Autodesk Inventor part; units mm, degrees
ref_plane "YZ Plane" through (0, 0, 0) normal (1, 0, 0) x (0, 1, 0)
ref_plane "XZ Plane" through (0, 0, 0) normal (0, 1, 0) x (-1, 0, 0)
ref_plane "XY Plane" through (0, 0, 0) normal (0, 0, 1) x (1, 0, 0)
sketch "Sketch1" plane through (0, 0, 0) normal (0, 0, 1) x (1, 0, 0)
  line L0 (-30, 30) -> (30, 30)
  line L1 (30, 30) -> (30, -30)
  line L2 (30, -30) -> (-30, -30)
  line L3 (-30, -30) -> (-30, 30)
  point P0 (0, 0)
  dimension "d0" = 60
  dimension "d1" = 60
  dimension "d2" = 30
  dimension "d3" = 30
extrude "Extrusion1" add sketch "Sketch1" along normal blind 2.6568
fillet "Fillet1" radius 2 2 edges at (30, -30, 1.3284) (-30, -30, 1.3284)
sketch "Sketch3" plane through (0, 0, 2.6568) normal (0, 0, 1) x (1, 0, 0)
  line L0 (-28, -30) -> (28, -30)
  line L1 (30, -28) -> (30, 30)
  line L2 (-30, 30) -> (-30, -28)
  line L3 (-15, -15) -> (-15, -25) construction
  line L4 (-17.75, -15) -> (-17.75, -25)
  line L5 (-12.25, -25) -> (-12.25, -15)
  arc A0 (-12.25, -15) -> (-17.75, -15) centre (-15, -15) ccw
  arc A1 (-17.75, -25) -> (-12.25, -25) centre (-15, -25) ccw
  line L6 (15, -15) -> (15, -25) construction
  line L7 (12.25, -15) -> (12.25, -25)
  line L8 (17.75, -25) -> (17.75, -15)
  arc A2 (17.75, -15) -> (12.25, -15) centre (15, -15) ccw
  arc A3 (12.25, -25) -> (17.75, -25) centre (15, -25) ccw
  point P0 (0, 0)
  point P1 (-15, -20)
  point P2 (15, -20)
  dimension "d14" = 10
  dimension "d15" = 5.5
  dimension "d16" = 5
  dimension "d17" = 15
  dimension "d18" = 5.5
  dimension "d19" = 45
  dimension "d20" = 10
  dimension "d21" = 5
extrude "Extrusion3" cut sketch "Sketch3" against normal through all
sketch "Sketch4" plane through (0, 0, 2.6568) normal (0, 0, 1) x (1, 0, 0)
  line L0 (30, -28) -> (30, 30)
  circle A0 centre (0, 9.85) radius 11
  line L1 (-28, -30) -> (28, -30)
  point P0 (0, 0)
  dimension "d24" = 22
  dimension "d25" = 30
  dimension "d31" = 39.85
extrude "Extrusion4" cut sketch "Sketch4" against normal blind 7
sketch "Sketch6" plane through (0, 0, 2.6568) normal (0, 0, 1) x (1, 0, 0)
  circle A0 centre (-15.5, -5.65) radius 1.75
  circle A1 centre (0, 9.85) radius 11
  point P0 (0, 0)
  dimension "d32" = 3.5
  dimension "d44" = 15.5
  dimension "d45" = 15.5
extrude "Extrusion6" cut sketch "Sketch6" against normal through all contours A0
pattern_linear "Rectangular Pattern1" count 2 spacing 31 along (1, 0, 0) count 2 spacing 31 along (0, 1, 0) of "Extrusion6"
fillet "Fillet2" radius 10 2 edges at (30, 30, 1.3284) (-30, 30, 1.3284)
properties part number "nema17_y_axis_motor_mount_12ga" material "UHMW, Black"
For this review, take the finished solid that the model builds, in its own axes (mm). A direction names the side the tool comes from. Give positions to 0.01 mm unless a question says otherwise; leave off trailing zeros. Loops run counter-clockwise (first coordinate to the right, second up) from the corner with the lowest first, then second, coordinate; pieces in that order, holes last.
Item 1: Take a section at C-C, the plane z = 0.8. State the section outline as (x, y) points.
Item 2: For line 1 along X through (y, z) = (-21, 0.8); line 2 along X through (y, z) = (-5, 0.5); line 3 along Y through (x, z) = (-15.5, 1.2), list the stretches that pass through material, from the lowest coordinate up.
Item 3: Draft analysis for pull direction X (two halves, no side actions). For faces 1 (the cylindrical face through (29.4, -29.43, 1.35)), 2 (the flat face through (6, 0, 2.657)), 3 (the cylindrical face through (-2.38, -0.89, 1.35)), state which applies: +X half, -X half, draft (parallel to the pull), parting line (faces both ways), or undercut.
Item 4: Take a section at A-A, the plane x = 0. State the section outline as (y, z) points.
Item 5: Take a section at B-B, the plane y = 9.85. State the section outline as (x, z) points.
Item 6: Take a section at D-D, the plane x = 15. State the section outline as (y, z) points.
Item 7: Tool access review of faces 4 (the flat face through (30, -4, 1)), 5 (the cylindrical face through (-14.94, -12.25, 1.35)): name each direction out of +Z, -Z, +X, -X, +Y, -Y from which nothing blocks a thin tool from reaching the whole face with its end or side.
Calculated:
1. outline: (-30, -28) arc R2 ccw to (-28, -30) - (28, -30) arc R2 ccw to (30, -28) - (30, 20) arc R10 ccw to (20, 30) - (-20, 30) arc R10 ccw to (-30, 20) - close; hole (-17.75, -25) arc R2.75 ccw to (-12.25, -25) - (-12.25, -15) arc R2.75 ccw to (-17.75, -15) - close; hole circle Ø3.5 at (-15.5, -5.65); hole circle Ø3.5 at (-15.5, 25.35); hole circle Ø22 at (0, 9.85); hole (12.25, -25) arc R2.75 ccw to (17.75, -25) - (17.75, -15) arc R2.75 ccw to (12.25, -15) - close; hole circle Ø3.5 at (15.5, -5.65); hole circle Ø3.5 at (15.5, 25.35)
2. line 1: x = -30 to -17.75, -12.25 to 12.25, 17.75 to 30
2. line 2: x = -30 to -17.12, -13.88 to 13.88, 17.12 to 30
2. line 3: y = -30 to -27.7, -12.3 to -7.4, -3.9 to 23.6, 27.1 to 30
3. face 1: +X half
3. face 2: draft
3. face 3: undercut
4. outline: (-30, 0) - (-1.15, 0) - (-1.15, 2.66) - (-30, 2.66) - close; (20.85, 0) - (30, 0) - (30, 2.66) - (20.85, 2.66) - close
5. outline: (-30, 0) - (-11, 0) - (-11, 2.66) - (-30, 2.66) - close; (11, 0) - (30, 0) - (30, 2.66) - (11, 2.66) - close
6. outline: (-30, 0) - (-27.75, 0) - (-27.75, 2.66) - (-30, 2.66) - close; (-12.25, 0) - (-7.33, 0) - (-7.33, 2.66) - (-12.25, 2.66) - close; (-3.97, 0) - (23.67, 0) - (23.67, 2.66) - (-3.97, 2.66) - close; (27.03, 0) - (30, 0) - (30, 2.66) - (27.03, 2.66) - close
7. face 4: +Z, -Z, +X, +Y, -Y
7. face 5: +Z, -Z
